```python
from build123d import *

# Parameters (mm, degrees)
SKETCH1_R           = 1.5
SKETCH1_R_2         = 3.815
BOSS_EXTRUDE1_DEPTH = 2.4
SKETCH2_W           = 25.5
SKETCH2_H           = 2.4
BOSS_EXTRUDE2_DEPTH = 35.8
CUT_EXTRUDE1_DEPTH  = 35.8
SKETCH4_R           = 3.8
SKETCH4_R_2         = 1.500976088
SKETCH4_R_3         = 1.5
CUT_EXTRUDE2_DEPTH  = 35.8


with BuildPart() as part:
    # Sketch1 → Boss-Extrude1 (new body)
    with BuildSketch(Plane.XY):
        with BuildLine():
            Line((0, 0), (25.5, 0))
            Line((25.5, 0), (25.5, 20))
            ThreePointArc((25.5, 20), (12.75, 30), (0, 20))
            Line((0, 20), (0, 0))
        make_face()
        with Locations((12.75, 24.571875)):
            Circle(SKETCH1_R, mode=Mode.SUBTRACT)
        with Locations((12.75, 16.871875)):
            Circle(SKETCH1_R_2, mode=Mode.SUBTRACT)
        with Locations((20.45, 16.871875)):
            Circle(SKETCH1_R, mode=Mode.SUBTRACT)
        with Locations((12.75, 9.171875)):
            Circle(SKETCH1_R, mode=Mode.SUBTRACT)
        with Locations((5.05, 16.871875)):
            Circle(SKETCH1_R, mode=Mode.SUBTRACT)
    extrude(amount=BOSS_EXTRUDE1_DEPTH)

    # Sketch2 → Boss-Extrude2 (add)
    with BuildSketch(Plane.XY.offset(2.4)):
        with Locations((12.75, 1.2)):
            Rectangle(SKETCH2_W, SKETCH2_H)
    extrude(amount=BOSS_EXTRUDE2_DEPTH)

    # Sketch3 → Cut-Extrude1 (cut)
    with BuildSketch(Plane.XZ):
        with BuildLine():
            ThreePointArc((0, 26.2), (3.514718626, 34.685281374), (12, 38.2))
            Line((12, 38.2), (0, 38.2))
            Line((0, 38.2), (0, 26.2))
        make_face()
        with BuildLine():
            Line((25.5, 38.2), (13.5, 38.2))
            ThreePointArc((13.5, 38.2), (21.985281374, 34.685281374), (25.5, 26.2))
            Line((25.5, 26.2), (25.5, 38.2))
        make_face()
    extrude(amount=-CUT_EXTRUDE1_DEPTH, mode=Mode.SUBTRACT)

    # Sketch4 → Cut-Extrude2 (cut)
    with BuildSketch(Plane.XZ):
        with Locations(Location((12.75, 26.823800226, 0), (0, 0, 270))):
            Circle(SKETCH4_R)
        with Locations(Location((5.89, 26.612165956, 0), (0, 0, 270))):
            Circle(SKETCH4_R_2)
        with Locations(Location((19.61, 26.612165956, 0), (0, 0, 270))):
            Circle(SKETCH4_R_3)
        with Locations(Location((12.75, 33.687165956, 0), (0, 0, 270))):
            Circle(SKETCH4_R_3)
        with Locations(Location((12.75, 20.037167493, 0), (0, 0, 270))):
            Circle(SKETCH4_R_3)
    extrude(amount=-CUT_EXTRUDE2_DEPTH, mode=Mode.SUBTRACT)


solid = part.part
```
Can you work these out from the model? Positions are in its coordinate system, mm. Round coordinates to 2 decimals unless told otherwise and drop trailing zeros. Loops run counter-clockwise (first coordinate to the right, second up) from the corner with the lowest first, then second, coordinate; pieces in that order, holes last. Notation, with made-up numbers: M 23.25,44.25 L 63.25,44.25 A18 ccw 63.25,59.25 Z; hole C -21,30.5 d8. An arc over 180 degrees is marked long. Answer as a JSON object with one key per item and string values. Group by question number.
Q1. Imagine slicing it at C-C, the plane x = 20.45. Please give me the cut outline in (y, z), then the cut area to 3 significant figures.
Q2. Imagine slicing it at B-B, the plane z = 19. Please give me the cut outline in (x, y).
Q3. Imagine slicing it at A-A, the plane x = 12.75. Count the separate pieces of the cut face and the enclosed holes in it, then the cut area to 3 significant figures.
Q4. Will these pins go through, and if not, where does the flat tip stop? pin 1 (5 mm diameter, centred on x = 7, y = 7.5, fed in from +Z); pin 2 (2 mm diameter, centred on x = 3, z = 33, fed in from +Y); pin 3 (12 mm diameter, centred on y = 6, z = 16, fed in from +X).
Q5. Please list where these lines run through material, in increasing order: L1, parallel to Y at x = 14.75, z = 9.5; L2, parallel to Y at x = 20.45, z = 1.05.
Q6. Imagine slicing it at D-D, the plane z = 3.5. Please give me the cut outline in (x, y), then the cut area to 3 significant figures.
Q7. We'd pull the mould along Y, two halves only. Please class faces 1 (the flat face through (13, 2.4, 16)), 2 (the cylindrical face through (12.92, 1.18, 30.62)), 3 (the flat face through (13, 0, 15)), 4 (the cylindrical face through (12.42, 7.71, 1.18)): +Y half, -Y half, draft (parallel to the pull), parting line (faces both ways), or undercut.
Findings:
{
 "1": {"outline": "M 0,0 L 15.37,0 L 15.37,2.4 L 2.4,2.4 L 2.4,25.37 L 0,25.37 Z; M 0,27.85 L 2.4,27.85 L 2.4,35.98 L 0,35.98 Z; M 18.37,0 L 27.5,0 L 27.5,2.4 L 18.37,2.4 Z", "area": "133 mm2"},
 "2": {"outline": "M 0,0 L 11.67,0 L 11.67,2.4 L 0,2.4 Z; M 13.83,0 L 25.5,0 L 25.5,2.4 L 13.83,2.4 Z"},
 "3": {"separate pieces": "7", "enclosed holes": "0", "area": "92.6 mm2"},
 "4": {"pin 1": "stops at z = 2.4", "pin 2": "stops at y = 2.4", "pin 3": "stops at x = 25.5"},
 "5": {"L1": "y = 0 to 2.4", "L2": "y = 0 to 15.37, 18.37 to 27.5"},
 "6": {"outline": "M 0,0 L 25.5,0 L 25.5,2.4 L 0,2.4 Z", "area": "61.2 mm2"},
 "7": {"face 1": "+Y half", "face 2": "draft", "face 3": "-Y half", "face 4": "undercut"}
}
